Input: part model. Units: mm. Frame: model coordinates. A direction names the side the tool comes from. Coordinates: 2 decimals unless noted, no trailing zeros. Loops run counter-clockwise (first coordinate to the right, second up) from the corner with the lowest first, then second, coordinate; pieces in that order, holes last.
Item 1: Reachability of faces 4 (the cylindrical face through (8.76, -1.19, 3.78)), 5 (the cylindrical face through (4.36, 30.995, -6.883)) from +Z, -Z, +X, -X, +Y, -Y: full face, straight path, thin tool, end or side. Return the list, or none.
Item 2: Section A-A on x = 7.5. Return loops of the section in (y, z), and give its area (3 significant figures).
Item 3: Pull-direction query (Y, two-part tool) for faces 1 (the cylindrical face through (5.86, -0.953, 3.026)), 2 (the flat face through (11.887, -2.3, -2.4)), 3 (the cylindrical face through (5.15, 4.65, -1.03)); classes: released by +Y, released by -Y, zero draft, split by the parting line, or undercut.
Item 4: Ray query, line 1 along X through (y, z) = (-24, -20.5); line 2 along Y through (x, z) = (6, 0); line 3 along Y through (x, z) = (4.5, 0). Return the intervals inside material, ascending.
Item 5: Contact query for flat-ended pins moving along their axis: P1, Ø19, axis at y = -10.5, z = -3.5, coming from the +X side; P2, Ø4, axis at x = 10, z = 0.5, coming from the +Y side; P3, Ø0.6, axis at x = 10, z = -3.5, coming from the -Y side; P4, Ø0.5, axis at y = 0, z = -3.5, coming from the +X side. Output: stop coordinate, or through.
Item 6: Section B-B on x = 2. Return loops of the section in (y, z).
```python
from build123d import *

# Parameters (mm, degrees)
SKETCH2_W               = 6.35
SKETCH2_H               = 0.8001
CUT_EXTRUDE1_SLOT_START = -5.715
CUT_EXTRUDE1_SLOT_DEPTH = 5.715
CIRPATTERN1_COUNT       = 4


with BuildPart() as part:
    # Sketch1 → Revolve1-MAIN BODY (revolve)
    with BuildSketch(Plane.XY, mode=Mode.PRIVATE) as revolve1_main_body_sk:
        with BuildLine():
            Line((0, 31.75), (0.79155417, 31.75))
            ThreePointArc((0.79155417, 31.75), (2.3749, 30.16665417), (3.95824583, 31.75))
            Line((3.95824583, 31.75), (4.7498, 31.75))
            Line((4.7498, 31.75), (4.7498, 4.7625))
            Line((4.7498, 4.7625), (11.8872, 4.7625))
            Line((11.8872, 4.7625), (11.8872, 3.17246))
            Line((11.8872, 3.17246), (0, 3.17246))
            Line((0, 3.17246), (0, 31.75))
        make_face()
    revolve(revolve1_main_body_sk.sketch.rotate(Axis((0, 0, 0), (1, 0, 0)), 90), axis=Axis((0, 0, 0), (1, 0, 0)))

    # Sketch2 → Cut-Revolve1-SLOT (revolve, cut)
    with BuildSketch(Plane.XY, mode=Mode.PRIVATE) as cut_revolve1_slot_sk:
        with Locations((8.7122, 4.36245)):
            Rectangle(SKETCH2_W, SKETCH2_H)
    revolve(cut_revolve1_slot_sk.sketch.rotate(Axis((0, 0, 0), (1, 0, 0)), 90), axis=Axis((0, 0, 0), (1, 0, 0)), mode=Mode.SUBTRACT)

    # Sketch3 → Cut-Extrude1-SLOT (cut)
    with BuildSketch(Plane(origin=(11.8872, 0, 0), x_dir=(0, 0, -1), z_dir=(1, 0, 0)).offset(CUT_EXTRUDE1_SLOT_START)):
        with BuildLine():
            Line((-0.3175, 3.949659164), (-0.3175, 3.156532306))
            ThreePointArc((-0.3175, 3.156532306), (0, 3.17246), (0.3175, 3.156532306))
            Line((0.3175, 3.156532306), (0.3175, 3.949659164))
            ThreePointArc((0.3175, 3.949659164), (0, 3.9624), (-0.3175, 3.949659164))
        make_face()
    cut_extrude1_slot = extrude(amount=CUT_EXTRUDE1_SLOT_DEPTH, mode=Mode.SUBTRACT)

    # CirPattern1: Cut-Extrude1-SLOT ×4 about axis
    cirpattern1_axis = Axis((0, 0, 0), (1, 0, 0))
    for i in range(1, CIRPATTERN1_COUNT):
        add(cut_extrude1_slot.rotate(cirpattern1_axis, i * 360 / CIRPATTERN1_COUNT), mode=Mode.SUBTRACT)


solid = part.part
```
Results found:
1. face 4: +X
1. face 5: +X, -X
2. outline: (-3.95, -0.32) arc R3.96 ccw to (-0.32, -3.95) - (-0.32, -3.16) arc R3.17 cw to (-3.16, -0.32) - close; (-3.95, 0.32) - (-3.16, 0.32) arc R3.17 cw to (-0.32, 3.16) - (-0.32, 3.95) arc R3.96 ccw to start; (0.32, -3.95) arc R3.96 ccw to (3.95, -0.32) - (3.16, -0.32) arc R3.17 cw to (0.32, -3.16) - close; (0.32, 3.16) arc R3.17 cw to (3.16, 0.32) - (3.95, 0.32) arc R3.96 ccw to (0.32, 3.95) - close
2. area: 15.7 mm2
3. face 1: undercut
3. face 2: zero draft
3. face 3: split by the parting line
4. line 1: x = 0 to 0.8, 3.95 to 4.75
4. line 2: y = -3.96 to -3.17, 3.17 to 3.96
4. line 3: y = -31.75 to -3.17, 3.17 to 31.75
5. P1: stops at x = 11.89
5. P2: stops at y = 3.95
5. P3: stops at y = -2.34
5. P4: stops at x = 6.17
6. outline: circle Ø60.42 at (0, 0); hole circle Ø6.34 at (0, 0)
